Autodesk Inventor part; units mm, degrees
ref_plane "YZ Plane" through (0, 0, 0) normal (1, 0, 0) x (0, 1, 0)
ref_plane "XZ Plane" through (0, 0, 0) normal (0, 1, 0) x (-1, 0, 0)
ref_plane "XY Plane" through (0, 0, 0) normal (0, 0, 1) x (1, 0, 0)
sketch "Sketch1" plane through (0, 0, 0) normal (0, 0, 1) x (1, 0, 0)
  arc A0 (0.2884, 3.0112) -> (0.2884, -3.0112) centre (0, 0) ccw
  arc A1 (15.7, -2.275) -> (15.7, 2.275) centre (15.7, 0) ccw
  line L0 (0, 3.025) -> (15.7, 2.275)
  line L1 (0, -3.025) -> (15.7, -2.275)
  dimension "d0" = 6.05
  dimension "d2" = 15.7
  dimension "d3" = 4.55
extrude "Extrusion1" add sketch "Sketch1" along normal blind 4 contours L0 A1 L1 A0
sketch "Sketch6" plane through (0, 0, 4) normal (0, 0, 1) x (1, 0, 0)
  arc A0 (0.6699, 9.9775) -> (2.6736, -9.636) centre (0, 0) ccw
  line L0 (0, 10) -> (24.986, 9.1622)
  line L1 (0, -10) -> (24.7714, -6.6271)
  line L2 (24.986, 9.1622) -> (54.986, -2.9102)
  line L3 (24.7714, -6.6271) -> (51.0332, -15.4223)
  line L4 (54.986, -2.9102) -> (51.0332, -15.4223)
  line L5 (15.7, 2.275) -> (0, 3.025)
  arc A1 (0, 3.025) -> (0, -3.025) centre (0, 0) ccw
  line L6 (0, -3.025) -> (15.7, -2.275)
  arc A2 (15.7, -2.275) -> (15.7, 2.275) centre (15.7, 0) ccw
  dimension "d32" = 20
  dimension "d33" = 25
  dimension "d34" = 25
  dimension "d37" = 160
  dimension "d39" = 30
  dimension "d56" = 51.0332
  dimension "d82" = 9.674
  dimension "d83" = 13.1217
  dimension "d84" = 153.73
extrude "Extrusion5" add sketch "Sketch6" against normal blind 4 contours L0 L2 L4 L3 L1 A0
sketch "Sketch8" plane through (0, 0, 4) normal (0, 0, 1) x (1, 0, 0)
  line L0 (0, -3.025) -> (15.7, -2.275)
  arc A0 (0.2884, 3.0112) -> (0.2884, -3.0112) centre (0, 0) ccw
  line L1 (0, 3.025) -> (15.7, 2.275)
  arc A1 (15.7, -2.275) -> (15.7, 2.275) centre (15.7, 0) ccw
extrude "Extrusion8" cut sketch "Sketch8" against normal blind 2.7 contours A0 L1 A1 L0
sketch "Sketch9" plane through (0, 0, 1.3) normal (0, 0, 1) x (1, 0, 0)
  line L0 (15.7, -2.275) -> (0, -3.025)
  circle A0 centre (0, 0) radius 3.025
  point P0 (0.2884, -3.0112)
extrude "Extrusion9" cut sketch "Sketch9" against normal through all
sketch "Sketch11" plane through (0, 0, 0) normal (0, 0, -1) x (-1, 0, 0)
  arc A0 (-48.1186, -3.7877) -> (-46.1454, -9.6796) centre (-47.4519, -6.8408) ccw
  arc A1 (-31.8422, -4.0122) -> (-33.2871, 0.3023) centre (-32.5646, -1.855) ccw
  line L0 (-53.146, -8.7478) -> (-23.9305, 1.0366) construction
  line L1 (-48.4443, -3.8776) -> (-33.2871, 0.3023)
  line L2 (-46.4595, -9.804) -> (-31.8422, -4.0122)
  line L3 (-54.986, -2.9102) -> (-51.0332, -15.4223)
  line L4 (-51.0332, -15.4223) -> (-24.7714, -6.6271)
  point P0 (0, 0)
  dimension "d60" = 6.25
  dimension "d64" = 4.55
  dimension "d65" = 3.125
  dimension "d66" = 2.275
  dimension "d74" = 6
  dimension "d75" = 7
  dimension "d77" = 15.7
fillet "Fillet3" radius 5 2 edges at (54.986, -2.9102, 2) (51.0332, -15.4223, 2)
extrude "Extrusion12" cut sketch "Sketch11" against normal blind 2.7 contours L1 A1 L2 A0
sketch "Sketch14" plane through (0, 0, 2.7) normal (0, 0, -1) x (-1, 0, 0)
  arc A0 (-48.4443, -3.8776) -> (-46.4595, -9.804) centre (-47.4519, -6.8408) ccw
  circle A1 centre (-47.4519, -6.8408) radius 3.125
  point P0 (0, 0)
  point P1 (-48.4443, -3.8776)
extrude "Extrusion13" cut sketch "Sketch14" against normal blind 2.7
properties part number "pata_superior_v3"
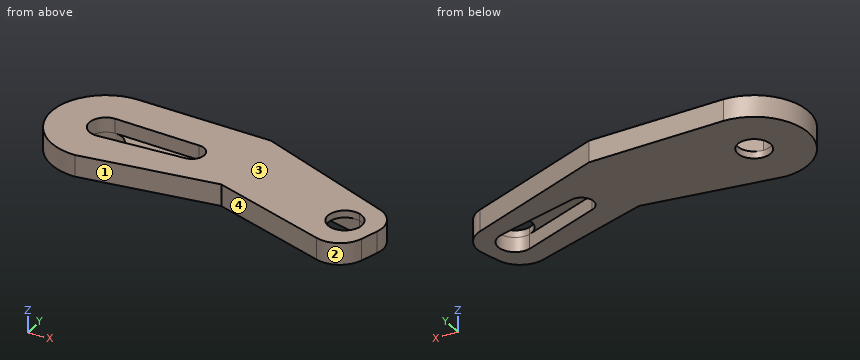
CAD build for the part. Positions are in the model's coordinates, mm. Face numbers are marked on the shaded views. Round coordinates to 2 decimals unless told otherwise and drop trailing zeros. Order: outer loops, then holes, each group sorted by start corner. A loop starts at its lowest first (then second) coordinate and runs counter-clockwise, first axis right, second up.
Item 1: Saw through at C-C on x = 36. Write the cut outline in (y, z).
Item 2: Saw through at A-A on x = -1. Write the cut outline in (y, z), then the cut area to 3 significant figures.
Item 3: Pin check, flat tips, straight feed: pin 1 (1 mm diameter, centred on y = 2, z = 3, fed in from -X); pin 2 (1 mm diameter, centred on x = 46, z = 3, fed in from +Y); pin 3 (1.5 mm diameter, centred on x = 0.5, z = 1.5, fed in from -Y). Stop position of each tip, or through.
Item 4: Probe line 1 along Y through (x, z) = (0, 0.35) (3 decimals); line 2 along Y through (x, z) = (1.5, 1.8); line 3 along Z through (x, y) = (32, -3). List the from-to ranges inside material, lowest first.
Item 5: Saw through at B-B on z = 1.9. State how many separate pieces and enclosed holes the cut face has, then the cut area to 3 significant figures.
Item 6: Mould opens along X. For the marked faces 1, 2, 3 and 4 say: pulls with the +X half, pulls with the -X half, needs draft (parallel to the pull), parting line crosses it, or undercut.
Item 7: Saw through at D-D on y = 4. Write the cut outline in (x, z).
Reported:
1. outline: (-10.39, 0) - (-5.66, 0) - (-5.66, 2.7) - (-0.45, 2.7) - (-0.45, 0) - (4.73, 0) - (4.73, 4) - (-10.39, 4) - close
2. outline: (-9.95, 0) - (-2.85, 0) - (-2.85, 4) - (-9.95, 4) - close; (2.85, 0) - (9.95, 0) - (9.95, 4) - (2.85, 4) - close
2. area: 56.8 mm2
3. pin 1: stops at x = -9.89
3. pin 2: stops at y = 0.91
3. pin 3: stops at y = -10
4. line 1: y = -10 to -3.025, 3.025 to 10
4. line 2: y = -9.8 to -2.95, 2.95 to 9.95
4. line 3: z = 2.7 to 4
5. separate pieces: 1
5. enclosed holes: 2
5. area: 798 mm2
6. face 1: undercut
6. face 2: parting line crosses it
6. face 3: needs draft
6. face 4: undercut
7. outline: (-9.17, 0) - (37.81, 0) - (37.81, 4) - (-9.17, 4) - close
